Autodesk Inventor part; units mm, degrees
ref_plane "YZ Plane" through (0, 0, 0) normal (1, 0, 0) x (0, 1, 0)
ref_plane "XZ Plane" through (0, 0, 0) normal (0, 1, 0) x (-1, 0, 0)
ref_plane "XY Plane" through (0, 0, 0) normal (0, 0, 1) x (1, 0, 0)
sketch "Sketch2" plane through (0, 0, 0) normal (0, 0, 1) x (1, 0, 0)
  line L0 (0, 0) -> (0, 35)
  line L1 (0, 35) -> (25, 35)
  line L2 (25, 35) -> (25, 27)
  line L3 (25, 27) -> (23, 27)
  line L4 (23, 27) -> (20, 0)
  line L5 (20, 0) -> (0, 0)
  dimension "d1" = 20
  dimension "d2" = 25
  dimension "d3" = 2
  dimension "d4" = 8
  dimension "d5" = 35
revolve "Revolution1" add sketch "Sketch2" angle 360 about axis through (0, 0, 0) along (0, 1, 0)
sketch "Sketch3" plane through (0, 35, 0) normal (0, 1, 0) x (1, 0, 0)
  circle A0 centre (0, 0) radius 25
  circle A1 centre (0, 0) radius 1
  dimension "d7" = 2
extrude "Extrusion1" cut sketch "Sketch3" against normal through all contours A1
sketch "Sketch4" plane through (0, 0, 0) normal (0, -1, 0) x (1, 0, 0)
  circle A0 centre (0, 0) radius 1
  circle A1 centre (0, 0) radius 20
  circle A2 centre (0, 0) radius 18
  dimension "d10" = 2
  dimension "potOpeningDia" = 36
extrude "Extrusion2" cut sketch "Sketch4" against normal blind 32 contours A2
sketch "Sketch5" plane through (0, 32, 0) normal (0, -1, 0) x (1, 0, 0)
  circle A0 centre (0, 0) radius 1
  circle A1 centre (0, 0) radius 18
  circle A2 centre (0, 0) radius 2.5
  dimension "d13" = 5
extrude "Extrusion3" add sketch "Sketch5" along normal blind 5 contours A2
sketch "Sketch6" plane through (0, 32, 0) normal (0, -1, 0) x (1, 0, 0)
  circle A0 centre (0, 0) radius 18
  circle A1 centre (0, 0) radius 5.5
  circle A2 centre (0, 0) radius 6.5
  dimension "d17" = 11
  dimension "d18" = 1
extrude "Extrusion4" add sketch "Sketch6" along normal blind 15 contours A2
properties part number "pot"
Source: CAD feature listing. Evaluate the final solid. Frame: model axes, mm. A direction names the side the tool comes from. Coordinates: 2 decimals unless noted, no trailing zeros. Loops run counter-clockwise (first coordinate to the right, second up) from the corner with the lowest first, then second, coordinate; pieces in that order, holes last. Notation, with made-up numbers: M 9,16.5 L 25,16.5 A14 ccw 25,20.5 Z; hole C 72.5,51 d4. An arc over 180 degrees is marked long. Answer in a Markdown table with one row per item.
Q1. Section D-D on y = 15.5. Return the cut outline in (x, z).
Answers below:
| item | result |
|---|---|
| outline | C 0,0 d43.44; hole C 0,0 d36 |
Q2. Draft query along Z for faces 3 (the flat face through (-18, 0, -3)), 4 (the flat face through (1, 27, -1)), 5 (the conical face through (-4.593, 10.689, 20.684)). Return one class per face: pulls with the +Z half, pulls with the -Z half, needs draft (parallel to the pull), parting line crosses it, or undercut.
Answers below:
| item | result |
|---|---|
| face 3 | needs draft |
| face 4 | undercut |
| face 5 | parting line crosses it |
Q3. First-contact query: pin 1 (3 mm diameter, centred on y = 22, z = -10.5, fed in from -X); pin 2 (1 mm diameter, centred on x = -7, z = -1.5, fed in from -Y); pin 3 (10 mm diameter, centred on y = 29, z = 18.5, fed in from -X). Flat tips, straight axial feed; report the tip coordinate or a pass-through.
Answers below:
| item | result |
|---|---|
| pin 1 | stops at x = -20.59 |
| pin 2 | stops at y = 32 |
| pin 3 | stops at x = -21.04 |
Q4. Section C-C on y = 22.5. Return the cut outline in (x, z), plus the area to 3 significant figures.
Answers below:
| item | result |
|---|---|
| outline | C 0,0 d45; C 0,0 d13; hole C 0,0 d36; hole C 0,0 d11 |
| area | 610 mm^2 |
Q5. Section B-B on z = 0. Return the cut outline in (x, y), plus the area to 3 significant figures.
Answers below:
| item | result |
|---|---|
| outline | M -25,27 L -23,27 L -20,0 L -18,0 L -18,32 L -6.5,32 L -6.5,17 L -5.5,17 L -5.5,32 L -2.5,32 L -2.5,27 L -1,27 L -1,35 L -25,35 Z; M 1,27 L 2.5,27 L 2.5,32 L 5.5,32 L 5.5,17 L 6.5,17 L 6.5,32 L 18,32 L 18,0 L 20,0 L 23,27 L 25,27 L 25,35 L 1,35 Z |
| area | 448 mm^2 |
Q6. Section A-A on x = 0. Return the cut outline in (y, z).
Answers below:
| item | result |
|---|---|
| outline | M 0,-20 L 27,-23 L 27,-25 L 35,-25 L 35,-1 L 27,-1 L 27,-2.5 L 32,-2.5 L 32,-5.5 L 17,-5.5 L 17,-6.5 L 32,-6.5 L 32,-18 L 0,-18 Z; M 0,18 L 32,18 L 32,6.5 L 17,6.5 L 17,5.5 L 32,5.5 L 32,2.5 L 27,2.5 L 27,1 L 35,1 L 35,25 L 27,25 L 27,23 L 0,20 Z |
Q7. Set-up query: faces 1 (the cylindrical face through (-0.54, 29.54, 2.44)), 2 (the flat face through (0, 35, 5)). Return all of +Z, -Z, +X, -X, +Y, -Y with unobstructed straight access to the full face (end or side cutting, diameter ignored); none if empty.
Answers below:
| item | result |
|---|---|
| face 1 | -Y |
| face 2 | +Z, -Z, +X, -X, +Y |
Q8. Ray query, probe 1 along Z at (x, y) = (-5, 25.5); probe 2 along Y at (x, z) = (-7, 8); probe 3 along X at (y, z) = (9.5, -7.5). Return the intervals inside material, ascending. Write a range as from..to.
Answers below:
| item | result |
|---|---|
| probe 1 | z = -22.28..-17.29, -4.15..-2.29, 2.29..4.15, 17.29..22.28 |
| probe 2 | y = 32..35 |
| probe 3 | x = -19.67..-16.36, 16.36..19.67 |
